Read the model definition and answer for the solid it produces. Units are mm, in the model's axes. A direction names the side the tool comes from. Round coordinates to 2 decimals unless told otherwise and drop trailing zeros. Order: outer loops, then holes, each group sorted by start corner. A loop starts at its lowest first (then second) coordinate and runs counter-clockwise, first axis right, second up. Notation, with made-up numbers: (34.5, 21) -> (87.5, 21) arc R9 cw to (87.5, 27) -> close; hole circle Ø11 at (66, 40.5). An arc over 180 degrees is marked (long way). Answer as a JSON object with one key per item and string values. Group by question number.
Item 1: Section C-C, the plane z = 7 is taken. Write down the section's boundary in (x, y).
Item 2: Given P1, Ø1.5, axis at y = 0, z = -12.5, coming from the -X side; P2, Ø1.5, axis at y = 0.5, z = -4.5, coming from the -X side; P3, Ø1.5, axis at y = -0.5, z = 5, coming from the -X side; P4, Ø1.5, axis at x = -2.5, z = 5.5, coming from the +Y side, each flat-ended and moving along its own axis, determine where each tip first touches the part or whether it passes through.
Item 3: The mould has two halves that part along Z. Classify faces 5 (the flat face through (-9.832, 0, 3)), 6 (the flat face through (-13, 0, -17)), 7 (the flat face through (-6, 1.5, 4)): pulls with the +Z half, pulls with the -Z half, needs draft (parallel to the pull), parting line crosses it, or undercut.
Item 4: Consider probe 1 along X at (y, z) = (1.4, 2.5); probe 2 along Z at (x, y) = (-10.5, -0.7); probe 3 along X at (y, z) = (0.3, -15). Determine where each line is inside the solid, lowest interval first. Write a range as from..to.
Item 5: Section B-B, the plane y = 1.05 is taken. Count the separate pieces of the cut face and the enclosed holes in it, plus the area to 3 significant figures.
Item 6: For faces 1 (the flat face through (-9.35, 0, -16)), 2 (the flat face through (15.25, 0, 0)), 3 (the flat face through (-26, 0, 9)), 4 (the cylindrical face through (9.36, 0.02, 4.5)), determine the directions among +Z, -Z, +X, -X, +Y, -Y from which every point of the face is accessible in a straight line to the end or side of a thin tool.
Item 7: Section A-A, the plane z = 16 is taken. Write down the section's boundary in (x, y).
Item 8: Section D-D, the plane x = 2.5 is taken. Write down the section's boundary in (y, z).
from build123d import *

# Parameters (mm, degrees)
SKETCH1_W           = 30.5
SKETCH1_H           = 34
BOSS_EXTRUDE1_DEPTH = 1.5
BOSS_EXTRUDE2_DEPTH = 3
SKETCH3_W           = 3
SKETCH3_H           = 8
SKETCH3_W_2         = 8
SKETCH3_H_2         = 3
BOSS_EXTRUDE3_DEPTH = 3
CUT_EXTRUDE1_DEPTH  = 4.0000001
CUT_EXTRUDE2_DEPTH  = 4.0000001
SKETCH6_W           = 8
SKETCH6_H           = 3
CUT_EXTRUDE3_DEPTH  = 4.0000001
CUT_EXTRUDE4_DEPTH  = 4.0000001
CUT_EXTRUDE6_DEPTH  = 4.0000001
SKETCH14_W          = 16.5
SKETCH14_H          = 9.25
CUT_EXTRUDE8_DEPTH  = 10
CUT_EXTRUDE10_DEPTH = 10
SKETCH18_R          = 5
CUT_EXTRUDE11_DEPTH = 10
SKETCH19_R          = 0.75
SKETCH19_W          = 4
SKETCH19_H          = 1.5
SKETCH19_W_2        = 1.5
SKETCH19_H_2        = 10
SKETCH19_H_3        = 7
CUT_EXTRUDE12_DEPTH = 10
SKETCH9_W           = 3
SKETCH9_H           = 4
BOSS_EXTRUDE4_DEPTH = 3


with BuildPart() as part:
    # Sketch1 → Boss-Extrude1 (new body, symmetric)
    with BuildSketch(Plane(origin=(0, 0, 0), x_dir=(1, 0, 0), z_dir=(0, 1, 0))):
        Rectangle(SKETCH1_W, SKETCH1_H)
    extrude(amount=BOSS_EXTRUDE1_DEPTH, both=True)

    # Sketch2 → Boss-Extrude2 (add)
    with BuildSketch(Plane(origin=(0, 1.5, 0), x_dir=(1, 0, 0), z_dir=(0, 1, 0))):
        with BuildLine():
            Line((-15.25, 17), (-24.07, 1.308996208))
            add(Edge.make_bspline(
                [(-24.07, 1.308996208), (-25.612124036, -1.43448158), (-30.226003395, -1.5229993), (-46.69780929, -11.088418218), (-55.382760657, -10.307171359), (-55.382760657, -17)],
                knots=[0, 0, 0, 0, 0.221130071, 0.603599568, 1, 1, 1, 1], degree=3))
            Line((-55.382760657, -17), (-15.25, -17))
            Line((-15.25, -17), (-15.25, 17))
        make_face()
    extrude(amount=-BOSS_EXTRUDE2_DEPTH)

    # Sketch3 → Boss-Extrude3 (add)
    with BuildSketch(Plane(origin=(0, 1.5, 0), x_dir=(1, 0, 0), z_dir=(0, 1, 0))):
        with Locations((16.75, 10)):
            Rectangle(SKETCH3_W, SKETCH3_H)
        with Locations((16.75, -10)):
            Rectangle(SKETCH3_W, SKETCH3_H)
        with Locations((-11.25, 18.5)):
            Rectangle(SKETCH3_W_2, SKETCH3_H_2)
        with Locations((11.25, 18.5)):
            Rectangle(SKETCH3_W_2, SKETCH3_H_2)
        with Locations((-51.382760657, -18.5)):
            Rectangle(SKETCH3_W_2, SKETCH3_H_2)
        with Locations((11.25, -18.5)):
            Rectangle(SKETCH3_W_2, SKETCH3_H_2)
        with Locations((-20.066380328, -18.5)):
            Rectangle(SKETCH3_W_2, SKETCH3_H_2)
    extrude(amount=-BOSS_EXTRUDE3_DEPTH)

    # Sketch4 → Cut-Extrude1 (cut, through all)
    with BuildSketch(Plane(origin=(0, 1.5, 0), x_dir=(1, 0, 0), z_dir=(0, 1, 0))):
        Polygon((-2.008190164, -14), (-2.008190164, -12.2), (-3.258190164, -12.2), (-3.258190164, -10), (-5.558190164, -10), (-5.558190164, -12.2), (-6.808190164, -12.2), (-6.808190164, -14), (-5.558190164, -14), (-5.558190164, -17), (-3.258190164, -17), (-3.258190164, -14), align=None)
        Polygon((-33.324570493, -14), (-33.324570493, -12.2), (-34.574570493, -12.2), (-34.574570493, -10), (-36.874570493, -10), (-36.874570493, -12.2), (-38.124570493, -12.2), (-38.124570493, -14), (-36.874570493, -14), (-36.874570493, -17), (-34.574570493, -17), (-34.574570493, -14), align=None)
    extrude(amount=-CUT_EXTRUDE1_DEPTH, mode=Mode.SUBTRACT)

    # Sketch5 → Cut-Extrude2 (cut, through all)
    with BuildSketch(Plane(origin=(0, 1.5, 0), x_dir=(1, 0, 0), z_dir=(0, 1, 0))):
        with BuildLine():
            Line((10.75, 20), (10.75, 7.75))
            ThreePointArc((10.75, 7.75), (2.5, -0.5), (-5.75, 7.75))
            Line((-5.75, 7.75), (-5.75, 20))
            Line((-5.75, 20), (10.75, 20))
        make_face()
    extrude(amount=-CUT_EXTRUDE2_DEPTH, mode=Mode.SUBTRACT)

    # Sketch6 → Cut-Extrude3 (cut, through all)
    with BuildSketch(Plane(origin=(0, 1.5, 0), x_dir=(1, 0, 0), z_dir=(0, 1, 0))):
        with Locations((-11.25, 18.5)):
            Rectangle(SKETCH6_W, SKETCH6_H)
    extrude(amount=-CUT_EXTRUDE3_DEPTH, mode=Mode.SUBTRACT)

    # Sketch7 → Cut-Extrude4 (cut, through all)
    with BuildSketch(Plane(origin=(0, 1.5, 0), x_dir=(1, 0, 0), z_dir=(0, 1, 0))):
        Polygon((-11.65, 17), (-9.35, 17), (-9.35, 14), (-8.1, 14), (-8.1, 12.2), (-9.35, 12.2), (-9.35, 10), (-11.65, 10), (-11.65, 12.2), (-12.9, 12.2), (-12.9, 14), (-11.65, 14), align=None)
    extrude(amount=-CUT_EXTRUDE4_DEPTH, mode=Mode.SUBTRACT)

    # Sketch8 → Cut-Extrude6 (cut, through all)
    with BuildSketch(Plane(origin=(0, 1.5, 0), x_dir=(1, 0, 0), z_dir=(0, 1, 0))):
        with BuildLine():
            Line((-24.066380328, -17), (-24.066380328, 1.315435696))
            Line((-24.066380328, 1.315435696), (-24.07, 1.308996208))
            add(Edge.make_bspline(
                [(-24.07, 1.308996208), (-25.612124036, -1.43448158), (-30.226003395, -1.5229993), (-46.69780929, -11.088418218), (-55.382760657, -10.307171359), (-55.382760657, -17)],
                knots=[0, 0, 0, 0, 0.221130071, 0.603599568, 1, 1, 1, 1], degree=3))
            Line((-55.382760657, -17), (-55.382760657, -20))
            Line((-55.382760657, -20), (-47.382760657, -20))
            Line((-47.382760657, -20), (-47.382760657, -17))
            Line((-47.382760657, -17), (-36.874570493, -17))
            Line((-36.874570493, -17), (-36.874570493, -14))
            Line((-36.874570493, -14), (-38.124570493, -14))
            Line((-38.124570493, -14), (-38.124570493, -12.2))
            Line((-38.124570493, -12.2), (-36.874570493, -12.2))
            Line((-36.874570493, -12.2), (-36.874570493, -10))
            Line((-36.874570493, -10), (-34.574570493, -10))
            Line((-34.574570493, -10), (-34.574570493, -12.2))
            Line((-34.574570493, -12.2), (-33.324570493, -12.2))
            Line((-33.324570493, -12.2), (-33.324570493, -14))
            Line((-33.324570493, -14), (-34.574570493, -14))
            Line((-34.574570493, -14), (-34.574570493, -17))
            Line((-34.574570493, -17), (-24.066380328, -17))
        make_face()
    extrude(amount=-CUT_EXTRUDE6_DEPTH, mode=Mode.SUBTRACT)

    # Sketch14 → Cut-Extrude8 (cut)
    with BuildSketch(Plane(origin=(0, 1.5, 0), x_dir=(1, 0, 0), z_dir=(0, 1, 0))):
        with Locations((2.691809836, -12.375)):
            Rectangle(SKETCH14_W, SKETCH14_H)
    extrude(amount=-CUT_EXTRUDE8_DEPTH, mode=Mode.SUBTRACT)

    # Sketch16 → Cut-Extrude10 (cut)
    with BuildSketch(Plane(origin=(0, 1.5, 0), x_dir=(1, 0, 0), z_dir=(0, 1, 0))):
        with BuildLine():
            Line((-5.558190164, -7.75), (2.691809836, -7.75))
            ThreePointArc((2.691809836, -7.75), (-1.433190164, -3.625), (-5.558190164, -7.75))
        make_face()
        with BuildLine():
            ThreePointArc((-5.558190164, -7.75), (-1.433190164, -11.875), (2.691809836, -7.75))
            Line((2.691809836, -7.75), (-5.558190164, -7.75))
        make_face()
        with BuildLine():
            Line((10.941809836, -7.75), (2.691809836, -7.75))
            ThreePointArc((2.691809836, -7.75), (6.816809836, -11.875), (10.941809836, -7.75))
        make_face()
        with BuildLine():
            ThreePointArc((10.941809836, -7.75), (6.816809836, -3.625), (2.691809836, -7.75))
            Line((2.691809836, -7.75), (10.941809836, -7.75))
        make_face()
    extrude(amount=-CUT_EXTRUDE10_DEPTH, mode=Mode.SUBTRACT)

    # Sketch18 → Cut-Extrude11 (cut)
    with BuildSketch(Plane(origin=(0, 1.5, 0), x_dir=(1, 0, 0), z_dir=(0, 1, 0))):
        with Locations((2.691809836, -7.75)):
            Circle(SKETCH18_R)
    extrude(amount=-CUT_EXTRUDE11_DEPTH, mode=Mode.SUBTRACT)

    # Sketch19 → Cut-Extrude12 (cut)
    with BuildSketch(Plane(origin=(0, 1.5, 0), x_dir=(1, 0, 0), z_dir=(0, 1, 0))):
        with Locations((-18.487833601, 0.912762829)):
            Circle(SKETCH19_R)
        with Locations((-11.831571961, -2.855782843)):
            Rectangle(SKETCH19_W, SKETCH19_H)
        with Locations((-15.694739931, -2.587237171)):
            Rectangle(SKETCH19_W_2, SKETCH19_H_2)
        with Locations((-11.881312648, 1.662762829)):
            Rectangle(SKETCH19_W, SKETCH19_H)
        with Locations((-11.831571961, -6.818375842)):
            Rectangle(SKETCH19_W, SKETCH19_H)
        with Locations((-18.487833601, -4.143833383)):
            Rectangle(SKETCH19_W_2, SKETCH19_H_3)
    extrude(amount=-CUT_EXTRUDE12_DEPTH, mode=Mode.SUBTRACT)

    # Sketch9 → Boss-Extrude4 (add)
    with BuildSketch(Plane(origin=(0, 1.5, 0), x_dir=(1, 0, 0), z_dir=(0, 1, 0))):
        with Locations((-25.566380328, -11)):
            Rectangle(SKETCH9_W, SKETCH9_H)
    extrude(amount=-BOSS_EXTRUDE4_DEPTH)


solid = part.part
Values found:
{
 "1": {"outline": "(-24.07, -1.5) -> (-19.24, -1.5) -> (-19.24, 1.5) -> (-24.07, 1.5) -> close; (-17.74, -1.5) -> (-16.44, -1.5) -> (-16.44, 1.5) -> (-17.74, 1.5) -> close; (-14.94, -1.5) -> (-13.83, -1.5) -> (-13.83, 1.5) -> (-14.94, 1.5) -> close; (-9.83, -1.5) -> (-5.49, -1.5) -> (-5.49, 1.5) -> (-9.83, 1.5) -> close; (10.87, -1.5) -> (18.25, -1.5) -> (18.25, 1.5) -> (10.87, 1.5) -> close"},
 "2": {"P1": "x = -18.2", "P2": "x = -22.7", "P3": "x = -24.07", "P4": "through"},
 "3": {"face 5": "undercut", "face 6": "pulls with the -Z half", "face 7": "needs draft"},
 "4": {"probe 1": "-24.07..-19.24, -17.74..-16.44, -14.94..-13.83, -9.83..15.25", "probe 2": "-10..-2.41, -0.91..2.11, 3.61..6.07, 7.57..17", "probe 3": "-16.37..-11.65, -9.35..-5.75, 10.75..15.25"},
 "5": {"separate pieces": "1", "enclosed holes": "6", "area": "845 mm2"},
 "6": {"face 1": "-Z, +Y, -Y", "face 2": "+X, +Y, -Y", "face 3": "-Z, -X, +Y, -Y", "face 4": "+Y, -Y"},
 "7": {"outline": "(-24.07, -1.5) -> (-5.56, -1.5) -> (-5.56, 1.5) -> (-24.07, 1.5) -> close; (10.94, -1.5) -> (15.25, -1.5) -> (15.25, 1.5) -> (10.94, 1.5) -> close"},
 "8": {"outline": "(-1.5, 0.5) -> (1.5, 0.5) -> (1.5, 2.75) -> (-1.5, 2.75) -> close"}
}
